The listing builds one solid part. Answer for the finished solid, in the listing's coordinates (mm). A direction names the side the tool comes from. Give positions to 0.01 mm unless a question says otherwise; leave off trailing zeros. Loops run counter-clockwise (first coordinate to the right, second up) from the corner with the lowest first, then second, coordinate; pieces in that order, holes last.
Item 1: Consider line 1 along Y through (x, z) = (-55, 1.2); line 2 along X through (y, z) = (2, 1.4); line 3 along Y through (x, z) = (-5, 1). Determine where each line is inside the solid, lowest interval first.
Item 2: A tool of negligible diameter and unlimited length cuts with its end or side. For faces 4 (the face through (58, -34, 1)), 5 (the face through (49.2, -22.5, 1)), from which of +Z, -Z, +X, -X, +Y, -Y can it reach the whole face along a straight path? Write none if from no direction.
Item 3: Section B-B, the plane y = 25 is taken. Give the vertices of the cut face in (x, z).
Item 4: The mould has two halves that part along X. Classify faces 1 (the face through (-22.5, 24.9, 1)), 2 (the face through (-1, -7, 2)), 3 (the face through (-59, -33, 1)): pulls with the +X half, pulls with the -X half, needs draft (parallel to the pull), parting line crosses it, or undercut.
Item 5: Section A-A, the plane x = -50 is taken. Give the vertices of the cut face in (y, z), and give its area (3 significant figures).
Item 6: Section D-D, the plane x = 0 is taken. Give the vertices of the cut face in (y, z).
Item 7: Section C-C, the plane z = 0.4 is taken. Give the number of separate pieces and of enclosed holes in the cut face, and give its area (3 significant figures).
from build123d import *

# Parameters (mm, degrees)
SKETCH1_R           = 1.6
BOSS_EXTRUDE1_DEPTH = 2


with BuildPart() as part:
    # Sketch1 → Boss-Extrude1 (new body)
    with BuildSketch(Plane.XY):
        with BuildLine():
            Line((55, 35), (-55, 35))
            ThreePointArc((-55, 35), (-58.535533906, 33.535533906), (-60, 30))
            Line((-60, 30), (-60, -30))
            ThreePointArc((-60, -30), (-58.535533906, -33.535533906), (-55, -35))
            Line((-55, -35), (55, -35))
            ThreePointArc((55, -35), (58.535533906, -33.535533906), (60, -30))
            Line((60, -30), (60, 30))
            ThreePointArc((60, 30), (58.535533906, 33.535533906), (55, 35))
        make_face()
        with Locations((-55, 30)):
            Circle(SKETCH1_R, mode=Mode.SUBTRACT)
        with Locations((-55, -30)):
            Circle(SKETCH1_R, mode=Mode.SUBTRACT)
        with Locations((55, -30)):
            Circle(SKETCH1_R, mode=Mode.SUBTRACT)
        with Locations((55, 30)):
            Circle(SKETCH1_R, mode=Mode.SUBTRACT)
        Circle(SKETCH1_R, mode=Mode.SUBTRACT)
        with BuildLine():
            Line((-20, 27.5), (20, 27.5))
            ThreePointArc((20, 27.5), (22.5, 25), (20, 22.5))
            Line((20, 22.5), (-20, 22.5))
            ThreePointArc((-20, 22.5), (-22.5, 25), (-20, 27.5))
        make_face(mode=Mode.SUBTRACT)
        with BuildLine():
            Line((-47.5, 20), (-47.5, -20))
            ThreePointArc((-47.5, -20), (-50, -22.5), (-52.5, -20))
            Line((-52.5, -20), (-52.5, 20))
            ThreePointArc((-52.5, 20), (-50, 22.5), (-47.5, 20))
        make_face(mode=Mode.SUBTRACT)
        with BuildLine():
            Line((-20, -23.636211525), (20, -23.636211525))
            ThreePointArc((20, -23.636211525), (22.5, -26.136211525), (20, -28.636211525))
            Line((20, -28.636211525), (-20, -28.636211525))
            ThreePointArc((-20, -28.636211525), (-22.5, -26.136211525), (-20, -23.636211525))
        make_face(mode=Mode.SUBTRACT)
        with BuildLine():
            Line((51.628871571, 20), (51.628871571, -20))
            ThreePointArc((51.628871571, -20), (49.128871571, -22.5), (46.628871571, -20))
            Line((46.628871571, -20), (46.628871571, 20))
            ThreePointArc((46.628871571, 20), (49.128871571, 22.5), (51.628871571, 20))
        make_face(mode=Mode.SUBTRACT)
    extrude(amount=BOSS_EXTRUDE1_DEPTH)


solid = part.part
Worked answers:
1. line 1: y = -35 to -31.6, -28.4 to 28.4, 31.6 to 35
1. line 2: x = -60 to -52.5, -47.5 to 46.63, 51.63 to 60
1. line 3: y = -35 to -28.64, -23.64 to 22.5, 27.5 to 35
2. face 4: +Z, -Z, +X, -Y
2. face 5: +Z, -Z
3. outline: (-60, 0) - (-22.5, 0) - (-22.5, 2) - (-60, 2) - close; (22.5, 0) - (60, 0) - (60, 2) - (22.5, 2) - close
4. face 1: undercut
4. face 2: needs draft
4. face 3: pulls with the -X half
5. outline: (-35, 0) - (-22.5, 0) - (-22.5, 2) - (-35, 2) - close; (22.5, 0) - (35, 0) - (35, 2) - (22.5, 2) - close
5. area: 50.0 mm2
6. outline: (-35, 0) - (-28.64, 0) - (-28.64, 2) - (-35, 2) - close; (-23.64, 0) - (-1.6, 0) - (-1.6, 2) - (-23.64, 2) - close; (1.6, 0) - (22.5, 0) - (22.5, 2) - (1.6, 2) - close; (27.5, 0) - (35, 0) - (35, 2) - (27.5, 2) - close
7. separate pieces: 1
7. enclosed holes: 9
7. area: 7,460 mm2
